from build123d import *

# Parameters (mm, degrees)
SKETCH1_W            = 225.4
SKETCH1_H            = 130.4
SKETCH1_W_2          = 200
SKETCH1_H_2          = 105
EXTRUSION1_DEPTH     = 40
EXTRUSION2_REACH     = 169.793
SKETCH2_W            = 200
SKETCH2_H            = 6.35
EXTRUSION4_DEPTH     = 137.206938149
SKETCH4_W            = 7.5
SKETCH4_H            = 5
EXTRUSION5_DEPTH     = 227.036125431
EXTRUSION6_REACH     = 228.036
SKETCH5_W            = 3
SKETCH5_H            = 3
SKETCH6_W            = 50.8
SKETCH6_H            = 3.175
EXTRUSION7_DEPTH     = 2.5
SKETCH7_W            = 25.4
SKETCH7_H            = 3.175
EXTRUSION8_DEPTH     = 22.86
EXTRUSION9_DEPTH     = 168.793265657
SKETCH20_W           = 12.7
SKETCH20_H           = 105
CUT_EXTRUDE425_DEPTH = 33.65
BOSS_EXTRUDE4_REACH  = 141.323
SKETCH21_W           = 5.0038
SKETCH21_H           = 12.7


with BuildPart() as part:
    # Sketch1 → Extrusion1 (new body)
    with BuildSketch(Plane.XY):
        Rectangle(SKETCH1_W, SKETCH1_H)
        Rectangle(SKETCH1_W_2, SKETCH1_H_2, mode=Mode.SUBTRACT)
    extrude(amount=-EXTRUSION1_DEPTH)

    # Sketch2 → Extrusion2 (add, up to next)
    with BuildSketch(Plane.XZ.offset(-52.5), mode=Mode.PRIVATE) as extrusion2_sk1:
        with Locations((0, -36.825)):
            Rectangle(SKETCH2_W, SKETCH2_H)
    extrusion2_tool1 = extrude(extrusion2_sk1.sketch, amount=EXTRUSION2_REACH, mode=Mode.PRIVATE) - part.part
    add(extrusion2_tool1.solids().sort_by_distance((0, 52.5, -36.825))[0])

    # Sketch3 → Extrusion4 (cut, through all)
    with BuildSketch(Plane(origin=(0, 0, -40), x_dir=(-1, 0, 0), z_dir=(0, 0, -1))):
        with BuildLine():
            Line((2.5, 43.2), (2.5, 39.530127019))
            ThreePointArc((2.5, 39.530127019), (0, 30.2), (-2.5, 39.530127019))
            Line((-2.5, 39.530127019), (-2.5, 43.2))
            ThreePointArc((-2.5, 43.2), (0, 45.7), (2.5, 43.2))
        make_face()
    extrude(amount=-EXTRUSION4_DEPTH, mode=Mode.SUBTRACT)

    # Sketch4 → Extrusion5 (cut, through all)
    with BuildSketch(Plane.ZY.offset(-100)):
        with Locations((-29.9, -50)):
            Rectangle(SKETCH4_W, SKETCH4_H)
    extrude(amount=-EXTRUSION5_DEPTH, mode=Mode.SUBTRACT)

    # Sketch5 → Extrusion6 (add, up to next)
    with BuildSketch(Plane(origin=(-100, 0, 0), x_dir=(0, 0, -1), z_dir=(1, 0, 0)), mode=Mode.PRIVATE) as extrusion6_sk1:
        with Locations((4, -51)):
            Rectangle(SKETCH5_W, SKETCH5_H)
    extrusion6_tool1 = extrude(extrusion6_sk1.sketch, amount=EXTRUSION6_REACH, mode=Mode.PRIVATE) - part.part
    add(extrusion6_tool1.solids().sort_by_distance((-100, -51, -4))[0])

    # Sketch6 → Extrusion7 (cut)
    with BuildSketch(Plane.XY):
        with Locations((0, -54.0875)):
            Rectangle(SKETCH6_W, SKETCH6_H)
    extrude(amount=-EXTRUSION7_DEPTH, mode=Mode.SUBTRACT)

    # Sketch7 → Extrusion8 (cut)
    with BuildSketch(Plane.XY):
        with Locations((-87.3, 54.0875)):
            Rectangle(SKETCH7_W, SKETCH7_H)
    extrusion8 = extrude(amount=-EXTRUSION8_DEPTH, mode=Mode.SUBTRACT)

    # Mirror1: Extrusion8 across plane
    add(extrusion8.mirror(Plane(origin=(0, 0, 0), x_dir=(0, 0, 1), z_dir=(1, 0, 0))), mode=Mode.SUBTRACT)

    # Sketch8 → Extrusion9 (cut, through all)
    with BuildSketch(Plane(origin=(0, -52.5, 0), x_dir=(-1, 0, 0), z_dir=(0, 1, 0))):
        Polygon((0, -33.65), (3.7465, -33.65), (3.7465, -28.6462), (-3.7465, -28.6462), (-3.7465, -33.65), align=None)
    extrude(amount=-EXTRUSION9_DEPTH, mode=Mode.SUBTRACT)

    # Sketch20 → Cut-Extrude425 (cut)
    with BuildSketch(Plane.XY):
        with Locations((-106.35, 0)):
            Rectangle(SKETCH20_W, SKETCH20_H)
        with Locations((106.35, 0)):
            Rectangle(SKETCH20_W, SKETCH20_H)
    extrude(amount=-CUT_EXTRUDE425_DEPTH, mode=Mode.SUBTRACT)

    # Sketch21 → Boss-Extrude4 (add, up to next)
    with BuildSketch(Plane(origin=(-3.7465, 0, 0), x_dir=(0, 0, -1), z_dir=(1, 0, 0)), mode=Mode.PRIVATE) as boss_extrude4_sk1:
        with Locations((31.1481, -58.85)):
            Rectangle(SKETCH21_W, SKETCH21_H)
    boss_extrude4_tool1 = extrude(boss_extrude4_sk1.sketch, amount=BOSS_EXTRUDE4_REACH, mode=Mode.PRIVATE) - part.part
    add(boss_extrude4_tool1.solids().sort_by_distance((-3.7465, -58.85, -31.1481))[0])


solid = part.part
Design review of the part built by this model. Coordinates are the model's own, in mm. A direction names the side the tool comes from. Give positions to 0.01 mm unless a question says otherwise; leave off trailing zeros. Loops run counter-clockwise (first coordinate to the right, second up) from the corner with the lowest first, then second, coordinate; pieces in that order, holes last. Notation, with made-up numbers: (49.25, 47) -> (84.25, 47) arc R30 ccw to (84.25, 72) -> close; hole circle Ø2 at (64, 13). An arc over 180 degrees is marked (long way). One line per question, with ' | ' between items. Start each with the question number.
(1) We need section B-B (z = -27). State the section outline as (x, y) points, and give its area (3 significant figures).
(2) We need section C-C (x = 0). State the section outline as (y, z) points (3 decimals).
(3) Draft analysis for pull direction Y (two halves, no side actions). For faces 1 (the face through (112.7, 0, -36)), 2 (the face through (-2, 65.2, -20)), 3 (the face through (-87, 55.675, -11)), state which applies: +Y half, -Y half, draft (parallel to the pull), parting line (faces both ways), or undercut.
(4) For line 1 (X direction, y = 35, z = -37); line 2 (Y direction, x = 78, z = -18) (3 decimals); line 3 (Y direction, x = 0, z = -37), list the stretches that pass through material, from the lowest coordinate up.
(5) We need section D-D (x = -94). State the section outline as (y, z) points (3 decimals), and give its area (3 significant figures).
(6) We need section A-A (y = 35.2). State the section outline as (x, z) points, and give its area (3 significant figures).
(7) For faces 4 (the face through (0.1, 45.7, -36.9)), 5 (the face through (-2, 52.5, -17)), 6 (the face through (87, 55.675, -11)), list the 3-axis set-ups (+Z, -Z, +X, -X, +Y, -Y) from which the entire face can be reached by the end or side of a thin tool; tool diameter is ignored.
(8) Insertion check: P1, Ø1, axis at x = -83, y = 53.5, coming from the +Z side; P2, Ø8, axis at x = 5.5, y = 46, coming from the +Z side; P3, Ø2, axis at x = 52.5, y = 38, coming from the +Z side. Each pin has a flat end and moves straight along its axis. Give the tip position at first contact, or say it passes through.
The answers:
1) outline: (-112.7, -65.2) -> (112.7, -65.2) -> (112.7, -52.5) -> (-112.7, -52.5) -> close; (-112.7, 52.5) -> (112.7, 52.5) -> (112.7, 65.2) -> (-112.7, 65.2) -> close | area: 5,730 mm^2
2) outline: (-65.2, -40) -> (30.2, -40) -> (30.2, -33.65) -> (-52.5, -33.65) -> (-52.5, -5.5) -> (-49.5, -5.5) -> (-49.5, -2.5) -> (-55.675, -2.5) -> (-55.675, 0) -> (-65.2, 0) -> close; (45.7, -40) -> (65.2, -40) -> (65.2, 0) -> (52.5, 0) -> (52.5, -33.65) -> (45.7, -33.65) -> close
3) face 1: draft | face 2: +Y half | face 3: undercut
4) line 1: x = -112.7 to -5, 5 to 112.7 | line 2: y = -65.2 to -52.5, 55.675 to 65.2 | line 3: y = -65.2 to 30.2, 45.7 to 65.2
5) outline: (-65.2, -40) -> (65.2, -40) -> (65.2, 0) -> (55.675, 0) -> (55.675, -22.86) -> (52.5, -22.86) -> (52.5, -33.65) -> (-52.5, -33.65) -> (-52.5, -5.5) -> (-49.5, -5.5) -> (-49.5, -2.5) -> (-52.5, -2.5) -> (-52.5, 0) -> (-65.2, 0) -> close | area: 1,620 mm^2
6) outline: (-112.7, -40) -> (-5, -40) -> (-5, -33.65) -> (-112.7, -33.65) -> close; (5, -40) -> (112.7, -40) -> (112.7, -33.65) -> (5, -33.65) -> close | area: 1,370 mm^2
7) face 4: +Z, -Z | face 5: +Z, +X, -X | face 6: +Z
8) P1: stops at z = -22.86 | P2: stops at z = -33.65 | P3: stops at z = -33.65
